Could you check a few things on this model? Use its own coordinates, in mm. A direction names the side the tool comes from. Round coordinates to 2 decimals unless told otherwise and drop trailing zeros. Loops run counter-clockwise (first coordinate to the right, second up) from the corner with the lowest first, then second, coordinate; pieces in that order, holes last.
from build123d import *

# Parameters (mm, degrees)
SKETCH_2_OUTSIDE_W  = 23.028
SKETCH_2_OUTSIDE_H  = 23.028
CUT_EXTRUDE_1_DEPTH = 32.560256653
CHAMFER_1_SIZE      = 0.5


with BuildPart() as part:
    # Эскиз1 → Повернуть1 (revolve)
    with BuildSketch(Plane.XY, mode=Mode.PRIVATE) as revolve_1_sk:
        Polygon((0, 0), (0, 5.7), (0.710140831, 6.93), (5, 6.93), (5, 4), (30, 4), (30, 0), align=None)
    revolve(revolve_1_sk.sketch.rotate(Axis((0, 0, 0), (1, 0, 0)), 90), axis=Axis((0, 0, 0), (1, 0, 0)))

    # Эскиз2 outside → Вырез-Вытянуть1 (cut, through all)
    with BuildSketch(Plane(origin=(0, 0, 0), x_dir=(0, 0, -1), z_dir=(1, 0, 0))):
        Rectangle(SKETCH_2_OUTSIDE_W, SKETCH_2_OUTSIDE_H)
        Polygon((6.92820323, 0), (3.464101615, 6), (-3.464101615, 6), (-6.92820323, 0), (-3.464101615, -6), (3.464101615, -6), align=None, mode=Mode.SUBTRACT)
    extrude(amount=CUT_EXTRUDE_1_DEPTH, mode=Mode.SUBTRACT)

    # Фаска1
    chamfer_1_edges = [part.edges().sort_by_distance(p)[0] for p in [
        (30, 0, -4),
    ]]
    chamfer(chamfer_1_edges, length=CHAMFER_1_SIZE)


solid = part.part
Item 1: If we section it at A-A, the plane z = 0: Please give me the cut outline in (x, y).
Results list:
outline: (0, -5.7) - (0.17, -6) - (5, -6) - (5, -4) - (29.5, -4) - (30, -3.5) - (30, 3.5) - (29.5, 4) - (5, 4) - (5, 6) - (0.17, 6) - (0, 5.7) - close
Item 2: Will these pins go through, and if not, where does the flat tip stop? pin 1 (1 mm diameter, centred on x = 24, y = 0.5, fed in from -Z); pin 2 (4 mm diameter, centred on y = 4.5, z = -4.5, fed in from +X); pin 3 (6 mm diameter, centred on x = 12.5, z = 2.5, fed in from +Y).
Results list:
pin 1: stops at z = -4
pin 2: stops at x = 5
pin 3: stops at y = 4
Item 3: If we section it at B-B, the plane x = 24: Please give me the cut outline in (y, z).
Results list:
outline: circle Ø8 at (0, 0)
Item 4: For faces 1 (the flat face through (5, -3, 3)), 2 (the flat face through (0, 0, 0)), which set-ups out of +Z, -Z, +X, -X, +Y, -Y let a thin tool reach every point of the face, with its end or its side?
Results list:
face 1: +X
face 2: +Z, -Z, -X, +Y, -Y
Item 5: If I drill on line 1 along X through (y, z) = (2.75, -3.5); line 2 along Y through (x, z) = (24.5, 0); line 3 along Z through (x, y) = (19.5, -3), over which ranges is the centre line in solid material (lowest first)?
Results list:
line 1: x = 0 to 5
line 2: y = -4 to 4
line 3: z = -2.65 to 2.65
